For this review, take the finished solid that the model builds, in its own axes (mm). Face numbers are marked on the shaded views. Round coordinates to 2 decimals unless told otherwise and drop trailing zeros. Write each loop counter-clockwise with the first axis right and the second up, starting at its lowest first coordinate (ties: lowest second). Pieces come first, ordered by that corner, then holes. Notation, with made-up numbers: M 22.5,69 L 71.5,69 A28 cw 71.5,88 Z; hole C 33.25,42.5 d5. An arc over 180 degrees is marked long. Answer in a Markdown table with one row per item.
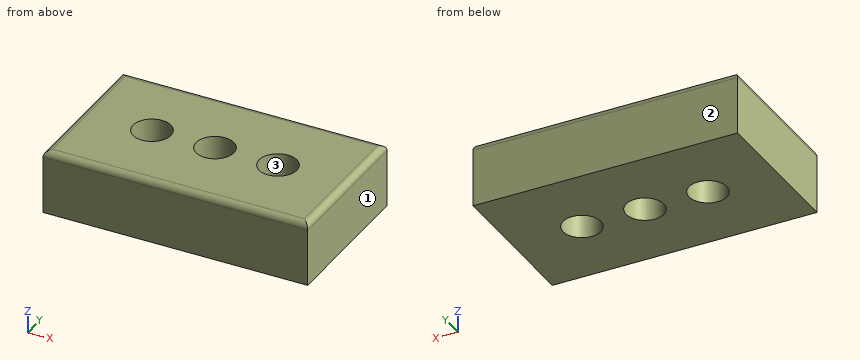
```python
from build123d import *

# Parameters (mm, degrees)
F0_W     = 105
F0_H     = 60
F0_R     = 7.5
F1_DEPTH = 20
F2_DEPTH = 25.4
F3_R     = 2.5


with BuildPart() as f1:
    # F0 (on Top) → F1 (new body)
    with BuildSketch(Plane.XY):
        Rectangle(F0_W, F0_H)
        with Locations((-25, 0)):
            Circle(F0_R, mode=Mode.SUBTRACT)
        with BuildLine():
            ThreePointArc((-7.5, 0), (0, 7.5), (7.5, 0))
            ThreePointArc((7.5, 0), (0, -7.5), (-7.5, 0))
        make_face(mode=Mode.SUBTRACT)
        with Locations((25, 0)):
            Circle(F0_R, mode=Mode.SUBTRACT)
    extrude(amount=F1_DEPTH)

    # F0 (on Top) → F2 (join)
    with BuildSketch(Plane.XY):
        Rectangle(F0_W, F0_H)
        with Locations((-25, 0)):
            Circle(F0_R, mode=Mode.SUBTRACT)
        with BuildLine():
            ThreePointArc((-7.5, 0), (0, 7.5), (7.5, 0))
            ThreePointArc((7.5, 0), (0, -7.5), (-7.5, 0))
        make_face(mode=Mode.SUBTRACT)
        with Locations((25, 0)):
            Circle(F0_R, mode=Mode.SUBTRACT)
    extrude(amount=F2_DEPTH)

    # F3
    f3_edges = [f1.edges().sort_by_distance(p)[0] for p in [
        (0, -30, 25.4),
        (-52.5, 0, 25.4),
        (0, 30, 25.4),
        (52.5, 0, 25.4),
    ]]
    fillet(f3_edges, radius=F3_R)


solid = f1.part
```
Q1. Mouldability with a two-part tool opening along X and no side actions: class the marked faces 1, 2 and 3 as +X half, -X half, draft (parallel to the pull), parting line (faces both ways), or undercut.
Found:
| item | result |
|---|---|
| face 1 | +X half |
| face 2 | draft |
| face 3 | undercut |
Q2. Take a section at A-A (x = 25). State the section outline as (y, z) points.
Found:
| item | result |
|---|---|
| outline | M -30,0 L -7.5,0 L -7.5,25.4 L -27.5,25.4 A2.5 ccw -30,22.9 Z; M 7.5,0 L 30,0 L 30,22.9 A2.5 ccw 27.5,25.4 L 7.5,25.4 Z |
Q3. Take a section at C-C (z = 21.25). State the section outline as (x, y) points, then the cut area to 3 significant figures.
Found:
| item | result |
|---|---|
| outline | M -52.5,-30 L 52.5,-30 L 52.5,30 L -52.5,30 Z; hole C -25,0 d15; hole C 0,0 d15; hole C 25,0 d15 |
| area | 5,770 mm² |
Q4. Take a section at D-D (x = -18.5). State the section outline as (y, z) points.
Found:
| item | result |
|---|---|
| outline | M -30,0 L -3.74,0 L -3.74,25.4 L -27.5,25.4 A2.5 ccw -30,22.9 Z; M 3.74,0 L 30,0 L 30,22.9 A2.5 ccw 27.5,25.4 L 3.74,25.4 Z |
Q5. For probe 1 along Y at (x, z) = (-25, 18.75); probe 2 along Y at (x, z) = (23.5, 12), list the stretches that pass through material, from the lowest coordinate up.
Found:
| item | result |
|---|---|
| probe 1 | -30 to -7.5, 7.5 to 30 |
| probe 2 | -30 to -7.35, 7.35 to 30 |
Q6. Take a section at B-B (y = 0). State the section outline as (x, z) points.
Found:
| item | result |
|---|---|
| outline | M -52.5,0 L -32.5,0 L -32.5,25.4 L -50,25.4 A2.5 ccw -52.5,22.9 Z; M -17.5,0 L -7.5,0 L -7.5,25.4 L -17.5,25.4 Z; M 7.5,0 L 17.5,0 L 17.5,25.4 L 7.5,25.4 Z; M 32.5,0 L 52.5,0 L 52.5,22.9 A2.5 ccw 50,25.4 L 32.5,25.4 Z |
